from build123d import *

# Parameters (mm, degrees)
F0_W           = 25
F0_H           = 12.5
F1_DEPTH       = 2
F2_W           = 2.0972218364
F2_H           = 12.5
F3_DEPTH       = 5
F4_W           = 12.5
F4_H           = 12.5694446266
F5_DEPTH       = 2
F6_SIZE        = 0.5
F8_D           = 2
F8_CSINK_D     = 3
F8_CSINK_ANGLE = 90
F9_DEPTH       = 0.1
F10_T4_DEPTH   = 13.4439057781
F10_T9_DEPTH   = 13.4439057781


# Not quite as in the source:
# - a fillet or chamfer that OpenCascade refuses, or shapes differently, is made with other operations: its cross-section is extruded or revolved along the edge and cut away or added


with BuildPart() as f1:
    # F0 (on Top) → F1 (new body)
    with BuildSketch(Plane.XY):
        Rectangle(F0_W, F0_H)
    extrude(amount=F1_DEPTH)

    # F2 (on face) → F3 (join)
    with BuildSketch(Plane.XY.offset(2)):
        with Locations((11.4513890818, 0)):
            Rectangle(F2_W, F2_H)
    extrude(amount=F3_DEPTH)

    # F4 (on face) → F5 (join)
    with BuildSketch(Plane.XY.offset(7)):
        with Locations((6.25, -0.0347223133)):
            Rectangle(F4_W, F4_H)
    extrude(amount=F5_DEPTH)

    # F6
    f6_edges = [f1.edges().sort_by_distance(p)[0] for p in [
        (10.402778, 6.25, 4.5),
        (-1.048611, 6.25, 2),
        (10.402778, -6.25, 4.5),
        (-1.048611, -6.25, 2),
        (5.201389, 6.25, 7),
    ]]
    chamfer(f6_edges, length=F6_SIZE)

    # F8 (through all)
    with Locations(Plane.XY.offset(2)):
        with Locations((-5.596134346, 0)):
            CounterSinkHole(F8_D / 2, F8_CSINK_D / 2, counter_sink_angle=F8_CSINK_ANGLE)

    # F9 (cut): a face of the model
    f9_faces = [f1.faces().sort_by_distance(p)[0] for p in [
        (6.25, -6.3194446266, 8),
    ]]
    extrude(f9_faces, amount=-F9_DEPTH, mode=Mode.SUBTRACT)

    # F10: chamfer of 0.5 on 1 edges, made by hand


with BuildPart() as f10_tool2:
    # F10_s3 → F10_t4 (new body)
    with BuildSketch(Plane.YZ.offset(-1.285841494)):
        Polygon((-5.7194446266, 7), (-6.2194446266, 7.5), (-6.2194446266, 7), align=None)
    extrude(amount=F10_T4_DEPTH)

    split(bisect_by=Plane(origin=(2.3263890818, 2.3263890818, 0), x_dir=(0, 0, 1), z_dir=(-0.7071067812, -0.7071067812, 0)), keep=Keep.TOP)


with BuildPart() as f1_1:
    add(f1.part)

    # F10_t1: cut F10_tool2
    add(f10_tool2.part, mode=Mode.SUBTRACT)


with BuildPart() as f10_tool7:
    # F10_s8 → F10_t9 (new body)
    with BuildSketch(Plane.YZ.offset(-1.285841494)):
        Polygon((-5.7194446266, 7), (-6.2194446266, 7.5), (-6.2194446266, 7), align=None)
    extrude(amount=F10_T9_DEPTH)

    split(bisect_by=Plane.YZ.offset(10.4027781636), keep=Keep.BOTTOM)


with BuildPart() as f1_2:
    add(f1_1.part)

    # F10_t6: cut F10_tool7
    add(f10_tool7.part, mode=Mode.SUBTRACT)


solid = f1_2.part
Build history of the part. All positions in model axes, mm. A direction names the side the tool comes from. Give positions to 0.01 mm unless a question says otherwise; leave off trailing zeros. Order: outer loops, then holes, each group sorted by start corner. A loop starts at its lowest first (then second) coordinate and runs counter-clockwise, first axis right, second up. Notation, with made-up numbers: M -14,69.25 L -10,69.25 A21 ccw -10,79.25 Z; hole C -24.75,-22.5 d1. An arc over 180 degrees is marked long. Put each result on its own line as item: value.
Item 1: Slice it at D-D, the plane z = 3.25. Write the cut outline in (x, y), plus the area to 3 significant figures.
From the geometry:
outline: M 10.4,-5.75 L 10.9,-6.25 L 12.5,-6.25 L 12.5,6.25 L 10.9,6.25 L 10.4,5.75 Z
area: 26.0 mm2
Item 2: Slice it at B-B, the plane y = 0. Write the cut outline in (x, z), plus the area to 3 significant figures.
From the geometry:
outline: M -12.5,0 L -6.6,0 L -6.6,1.5 L -7.1,2 L -12.5,2 Z; M -4.6,0 L 12.5,0 L 12.5,9 L 0,9 L 0,7 L 10.4,7 L 10.4,2 L -4.1,2 L -4.6,1.5 Z
area: 81.2 mm2
Item 3: Probe line 1 (Z direction, x = 3.75, y = -5); line 2 (X direction, y = 0, z = 0.75); line 3 (X direction, y = 2.5, z = 3.5). List the from-to ranges inside material, lowest first. Write a range as [from, to].
From the geometry:
line 1: z = [0, 2], [7, 9]
line 2: x = [-12.5, -6.6], [-4.6, 12.5]
line 3: x = [10.4, 12.5]
Item 4: 3-axis set-ups, long thin cutter, end or side, ignore diameter. For faces 5 (the flat face through (10.403, 0, 4)), 6 (the flat face through (0, 0, 8)), 7 (the flat face through (-12.5, 0, 1)), 8 (the flat face through (6, -6.219, 8)), 9 (the cylindrical face through (-6.52, -0.38, 0.74)): which of +Z, -Z, +X, -X, +Y, -Y reach the whole face in a straight line?
From the geometry:
face 5: -X, +Y, -Y
face 6: +Z, -X, +Y, -Y
face 7: +Z, -Z, -X, +Y, -Y
face 8: +Z, +X, -X, -Y
face 9: +Z, -Z
Item 5: Flat gauge pins, fed straight in: pin 1 Ø2.5 at (x, y) = (-5.6, 0) entering from +Z; pin 2 Ø1.5 at (x, z) = (-9.5, 2.5) entering from +Y; pin 3 Ø0.6 at (x, z) = (3.5, 8.5) entering from -Y; pin 4 Ø3 at (x, y) = (5, 2.5) entering from -Z. Where does each tip first touch, or does it go through?
From the geometry:
pin 1: stops at z = 1.75
pin 2: stops at y = 6
pin 3: stops at y = -6.22
pin 4: stops at z = 0
Item 6: Slice it at C-C, the plane x = -9. Write the cut outline in (y, z).
From the geometry:
outline: M -6.25,0 L 6.25,0 L 6.25,1.5 L 5.75,2 L -5.75,2 L -6.25,1.5 Z
Item 7: Slice it at A-A, the plane x = 6. Write the cut outline in (y, z), plus the area to 3 significant figures.
From the geometry:
outline: M -6.25,0 L 6.25,0 L 6.25,1.5 L 5.75,2 L -5.75,2 L -6.25,1.5 Z; M -6.22,7.5 L -5.72,7 L 5.75,7 L 6.25,7.5 L 6.25,9 L -6.22,9 Z
area: 49.4 mm2
Item 8: Two-plate mould, pull along Z, no slides. Class faces 1 (the flat face through (6, 0, 9)), 2 (the flat face through (0, 0, 0)), 3 (the flat face through (5, 0, 7)), 4 (the flat face through (3, 6.25, 1)): +Z half, -Z half, draft (parallel to the pull), parting line (faces both ways), or undercut.
From the geometry:
face 1: +Z half
face 2: -Z half
face 3: undercut
face 4: draft
